Answer from the drawing. Dimensions are ordinates in mm from the lowest x, y and z of the part. A direction names the side the tool comes from. Coordinates: 2 decimals unless noted, no trailing zeros. Write each loop counter-clockwise with the first axis right and the second up, starting at its lowest first coordinate (ties: lowest second). Pieces come first, ordered by that corner, then holes. Notation, with made-up numbers: (-9, 53.25) - (38, 53.25) arc R11 cw to (38, 57.25) - close; hole circle Ø6 at (42, 41.25). An arc over 180 degrees is marked (long way). Answer as a JSON object with one key per item and string values. Group by question number.
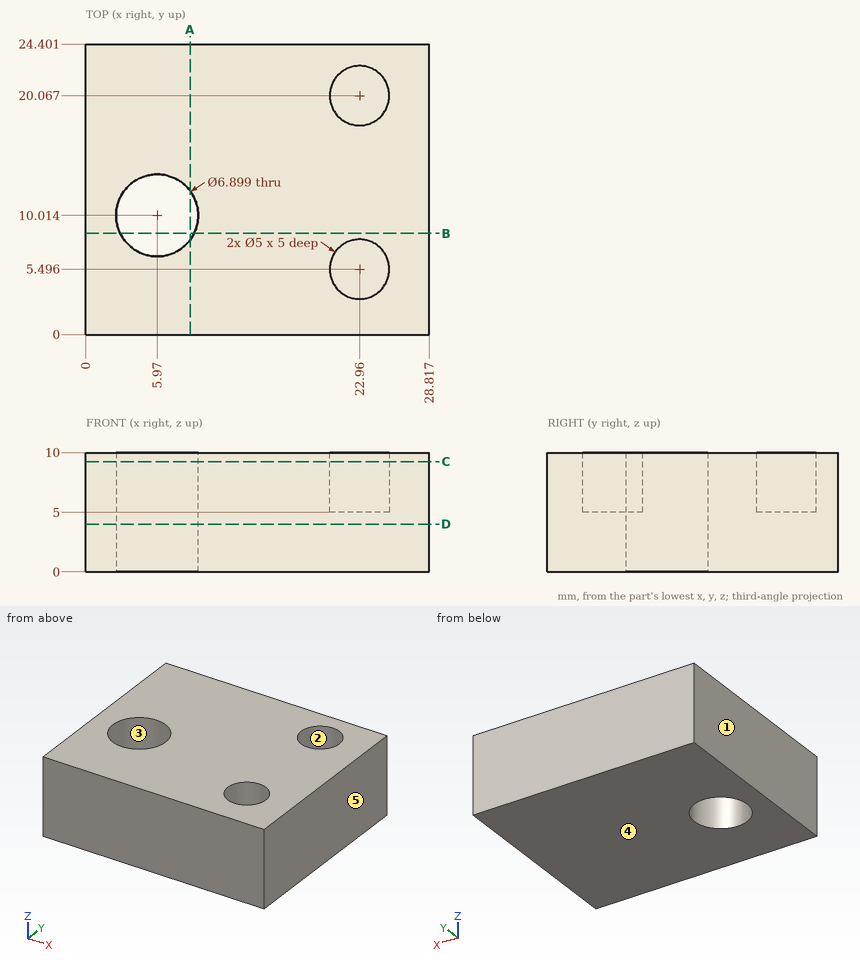
Q1. A tool of negligible diameter and unlimited length cuts with its end or side. For the marked faces 1 and 2, from which of +Z, -Z, +X, -X, +Y, -Y can it reach the whole face along a straight path? Write none if from no direction.
Q2. For a pull along X with two mould halves and no side action, classify the marked faces 3, 4 and 5 as +X half, -X half, draft (parallel to the pull), parting line (faces both ways), or undercut.
Q3. Consider L1, parallel to Y at x = 23, z = 5.25 (1 decimal); L2, parallel to X at y = 10.75, z = 2; L3, parallel to Y at x = 8.5, z = 4.25. Determine where each line is inside the solid, lowest interval first. Write a range as from..to.
Q4. Section A-A on x = 8.75 is taken. Determine the outline of the cut face in (y, z), plus the area to 3 significant figures.
Q5. Flat-ended cylindrical pins translate along their axes: pin 1 Ø4.5 at (x, y) = (22.96, 5.5) entering from +Z; pin 2 Ø4 at (x, y) = (5.97, 10.01) entering from +Z. Find the tip coordinate at first contact, or state that the pin passes through.
Q6. Section C-C on z = 9.25 is taken. Count the separate pieces of the cut face and the enclosed holes in it.
Q7. Section B-B on y = 8.5 is taken. Determine the outline of the cut face in (x, z), plus the area to 3 significant figures.
Q8. Section D-D on z = 4 is taken. Determine the outline of the cut face in (x, y).
Numbers:
{
 "1": {"face 1": "+Z, -Z, -X, +Y, -Y", "face 2": "+Z"},
 "2": {"face 3": "undercut", "face 4": "draft", "face 5": "+X half"},
 "3": {"L1": "y = 0..3, 8..17.6, 22.6..24.4", "L2": "x = 0..2.6, 9.34..28.82", "L3": "y = 0..7.67, 12.36..24.4"},
 "4": {"outline": "(0, 0) - (7.97, 0) - (7.97, 10) - (0, 10) - close; (12.06, 0) - (24.4, 0) - (24.4, 10) - (12.06, 10) - close", "area": "203 mm²"},
 "5": {"pin 1": "stops at z = 5", "pin 2": "passes through"},
 "6": {"separate pieces": "1", "enclosed holes": "3"},
 "7": {"outline": "(0, 0) - (2.87, 0) - (2.87, 10) - (0, 10) - close; (9.07, 0) - (28.82, 0) - (28.82, 10) - (9.07, 10) - close", "area": "226 mm²"},
 "8": {"outline": "(0, 0) - (28.82, 0) - (28.82, 24.4) - (0, 24.4) - close; hole circle Ø6.9 at (5.97, 10.01)"}
}
